Can you work these out from the drawing? Everything is in mm from the part's minimum corner. A direction names the side the tool comes from. Round coordinates to 2 decimals unless told otherwise and drop trailing zeros. Write each loop counter-clockwise with the first axis right and the second up, starting at its lowest first coordinate (ties: lowest second). Pieces come first, ordered by that corner, then holes. Notation, with made-up numbers: M 48,-12 L 81,-12 A11 ccw 81,-2 Z; hole C -6,-17.5 d2. An arc over 180 degrees is marked long. Use a Markdown table: item, result. Add a question column.
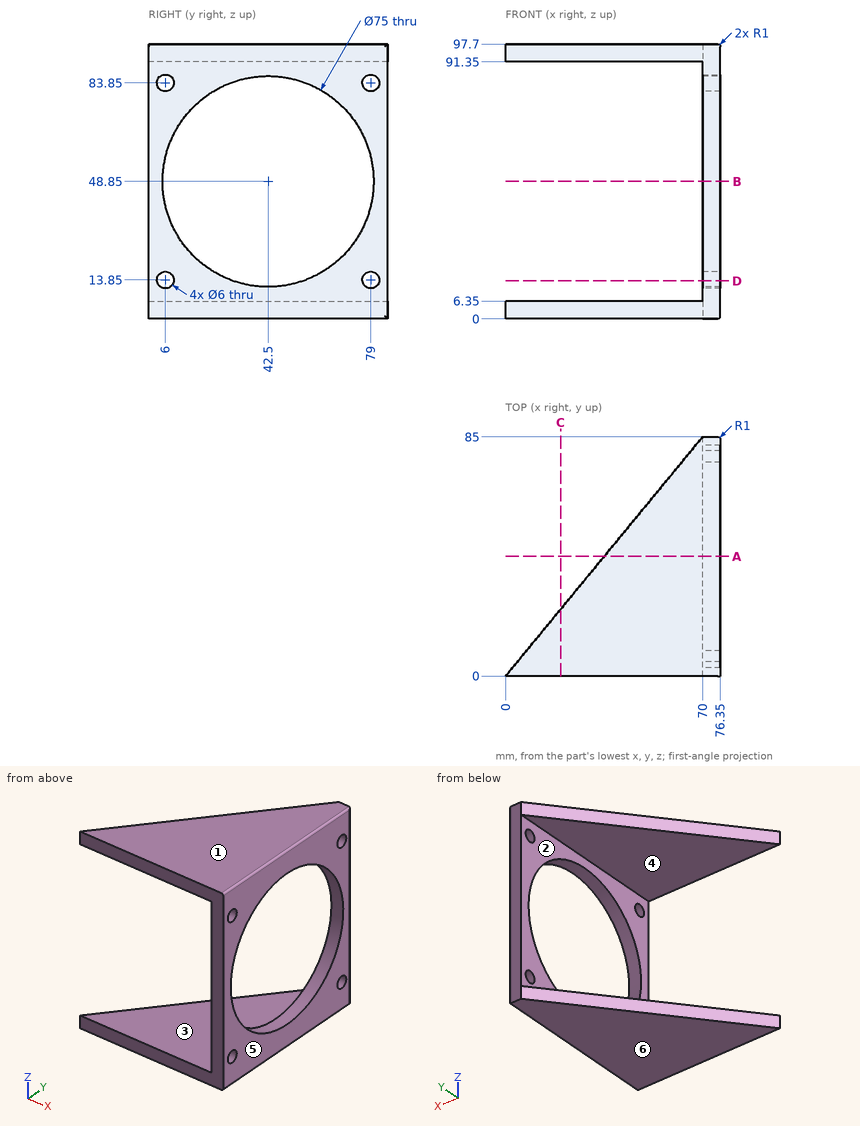
Item 1: On a 3-axis mill with a long thin cutter (end or side, diameter ignored), from which of +Z, -Z, +X, -X, +Y, -Y can I reach the whole of each face in a straight line? I mean the marked faces 1 and 2. Say none if no direction works.
Item 2: If we mould it in two halves opening along Z, with no side actions, what happens to the marked faces 3, 4, 5 and 6? For each: +Z half, -Z half, draft (parallel to the pull), parting line (faces both ways), or undercut.
Item 3: I need wall thicknesses on probe 1 along Z at (x, y) = (38, 37); probe 2 along Y at (x, z) = (73.25, 48.85); probe 3 along X at (y, z) = (10, 87.5). Which ranges of each line are inside material? Lowest first, please. Write a range as from..to.
Item 4: Imagine slicing it at B-B on z = 48.85. List the corners of the cut face in (x, y) for me, plus the area to 3 significant figures.
Item 5: Imagine slicing it at D-D on z = 13.5. List the corners of the cut face in (x, y) for me, plus the area to 3 significant figures.
Item 6: Imagine slicing it at A-A on y = 42.5. List the corners of the cut face in (x, z) for me.
Item 7: For pin 1 Ø9.5 at (y, z) = (6, 83.85) entering from -X, with a flat end and sliding along its axis, tell me the tip position at first contact or that it passes through.
Item 8: Imagine slicing it at C-C on x = 19.5. List the corners of the cut face in (y, z) for me, plus the area to 3 significant figures.
The answers:
| question | item | result |
|---|---|---|
| 1 | face 1 | +Z, +X, -X, +Y, -Y |
| 1 | face 2 | -X, +Y, -Y |
| 2 | face 3 | undercut |
| 2 | face 4 | undercut |
| 2 | face 5 | draft |
| 2 | face 6 | -Z half |
| 3 | probe 1 | 0..6.35, 91.35..97.7 |
| 3 | probe 2 | 0..5, 80..85 |
| 3 | probe 3 | 70..76.35 |
| 4 | outline | M 70,0 L 76.35,0 L 76.35,5 L 70,5 Z; M 70,80 L 76.35,80 L 76.35,84 A1 ccw 75.35,85 L 70,85 Z |
| 4 | area | 63.3 mm² |
| 5 | outline | M 70,0 L 76.35,0 L 76.35,3.02 L 70,3.02 Z; M 70,8.98 L 76.35,8.98 L 76.35,29.98 L 70,29.98 Z; M 70,55.02 L 76.35,55.02 L 76.35,76.02 L 70,76.02 Z; M 70,81.98 L 76.35,81.98 L 76.35,84 A1 ccw 75.35,85 L 70,85 Z |
| 5 | area | 305 mm² |
| 6 | outline | M 35,0 L 75.35,0 A1 ccw 76.35,1 L 76.35,11.35 L 70,11.35 L 70,6.35 L 35,6.35 Z; M 35,91.35 L 70,91.35 L 70,86.35 L 76.35,86.35 L 76.35,96.7 A1 ccw 75.35,97.7 L 35,97.7 Z |
| 7 | pin 1 | x = 70 |
| 8 | outline | M 0,0 L 23.68,0 L 23.68,6.35 L 0,6.35 Z; M 0,91.35 L 23.68,91.35 L 23.68,97.7 L 0,97.7 Z |
| 8 | area | 301 mm² |
